Model file for the job. Use its own axes, mm. A direction names the side the tool comes from. Round coordinates to 2 decimals unless told otherwise and drop trailing zeros. Loops run counter-clockwise (first coordinate to the right, second up) from the corner with the lowest first, then second, coordinate; pieces in that order, holes last. Notation, with made-up numbers: (-7.75, -35) - (44.25, -35) arc R24 cw to (44.25, 0) - close; hole circle Ø7 at (81, 4.5). An arc over 180 degrees is marked (long way). Answer as a JSON object with one key per item and string values.
from build123d import *

# Parameters (mm, degrees)
RESSALTO_EXTRUS_O1_DEPTH = 65
ESBO_O2_W                = 40
ESBO_O2_H                = 40
RESSALTO_EXTRUS_O2_DEPTH = 4
ESBO_O4_W                = 5
ESBO_O4_H                = 5
RESSALTO_EXTRUS_O3_DEPTH = 13.5
ESBO_O5_W                = 40
ESBO_O5_H                = 40
ESBO_O5_W_2              = 30
ESBO_O5_H_2              = 30
RESSALTO_EXTRUS_O4_DEPTH = 4


with BuildPart() as part:
    # Esboço1 → Ressalto-extrusão1 (new body)
    with BuildSketch(Plane.XY):
        with BuildLine():
            Line((18, 0), (20, 0))
            Line((20, 0), (20, 40))
            Line((20, 40), (-20, 40))
            Line((-20, 40), (-20, 0))
            Line((-20, 0), (-18, 0))
            Line((-18, 0), (-18, 9))
            Line((-18, 9), (-18, 27))
            ThreePointArc((-18, 27), (-15.363961031, 33.363961031), (-9, 36))
            Line((-9, 36), (9, 36))
            ThreePointArc((9, 36), (15.363961031, 33.363961031), (18, 27))
            Line((18, 27), (18, 0))
        make_face()
    extrude(amount=RESSALTO_EXTRUS_O1_DEPTH)

    # Esboço2 → Ressalto-extrusão2 (add)
    with BuildSketch(Plane(origin=(0, 0, 0), x_dir=(-1, 0, 0), z_dir=(0, 0, -1))):
        with Locations((0, 20)):
            Rectangle(ESBO_O2_W, ESBO_O2_H)
        with BuildLine():
            Line((-5, 30), (-5, 6))
            ThreePointArc((-5, 6), (-9, 2), (-13, 6))
            Line((-13, 6), (-13, 30))
            ThreePointArc((-13, 30), (-9, 34), (-5, 30))
        make_face(mode=Mode.SUBTRACT)
        with BuildLine():
            Line((13, 30), (13, 6.321034479))
            ThreePointArc((13, 6.321034479), (9, 2.321034479), (5, 6.321034479))
            Line((5, 6.321034479), (5, 30))
            ThreePointArc((5, 30), (9, 34), (13, 30))
        make_face(mode=Mode.SUBTRACT)
    ressalto_extrus_o2 = extrude(amount=RESSALTO_EXTRUS_O2_DEPTH)

    # Esboço4 → Ressalto-extrusão3 (add)
    with BuildSketch(Plane(origin=(0, 0, -4), x_dir=(-1, 0, 0), z_dir=(0, 0, -1))):
        with Locations((17.5, 37.5)):
            Rectangle(ESBO_O4_W, ESBO_O4_H)
        with Locations((17.5, 2.5)):
            Rectangle(ESBO_O4_W, ESBO_O4_H)
        with Locations((-17.5, 37.5)):
            Rectangle(ESBO_O4_W, ESBO_O4_H)
        with Locations((-17.5, 2.5)):
            Rectangle(ESBO_O4_W, ESBO_O4_H)
    ressalto_extrus_o3 = extrude(amount=RESSALTO_EXTRUS_O3_DEPTH)

    # Esboço5 → Ressalto-extrusão4 (add)
    with BuildSketch(Plane(origin=(0, 0, -17.5), x_dir=(-1, 0, 0), z_dir=(0, 0, -1))):
        with Locations((0, 20)):
            Rectangle(ESBO_O5_W, ESBO_O5_H)
        with Locations((0, 20)):
            Rectangle(ESBO_O5_W_2, ESBO_O5_H_2, mode=Mode.SUBTRACT)
    ressalto_extrus_o4 = extrude(amount=RESSALTO_EXTRUS_O4_DEPTH)

    # Espelhar1: Ressalto-extrusão2, Ressalto-extrusão3, Ressalto-extrusão4 across plane
    add(ressalto_extrus_o2.mirror(Plane.XY.offset(32.5)))
    add(ressalto_extrus_o3.mirror(Plane.XY.offset(32.5)))
    add(ressalto_extrus_o4.mirror(Plane.XY.offset(32.5)))


solid = part.part
1) Tool access for faces 1 (the cylindrical face through (9, 34, 67)), 2 (the flat face through (0, 3, -17.5)), 3 (the flat face through (18, 14, 32)), 4 (the flat face through (-17, 35, 76)): list every direction of +Z, -Z, +X, -X, +Y, -Y with a clear straight run to the whole face (end or side of a thin tool).
Values follow:
{"face 1": "+Z, -Z", "face 2": "+Y, -Y", "face 3": "-Y", "face 4": "+X, -X"}
2) Slice it at C-C on x = -4. List the corners of the cut face in (y, z).
Values follow:
{"outline": "(0, -21.5) - (5, -21.5) - (5, -17.5) - (0, -17.5) - close; (0, -4) - (40, -4) - (40, 69) - (0, 69) - (0, 65) - (36, 65) - (36, 0) - (0, 0) - close; (0, 82.5) - (5, 82.5) - (5, 86.5) - (0, 86.5) - close; (35, -21.5) - (40, -21.5) - (40, -17.5) - (35, -17.5) - close; (35, 82.5) - (40, 82.5) - (40, 86.5) - (35, 86.5) - close"}
3) Slice it at D-D on z = 39. List the corners of the cut face in (x, y).
Values follow:
{"outline": "(-20, 0) - (-18, 0) - (-18, 27) arc R9 cw to (-9, 36) - (9, 36) arc R9 cw to (18, 27) - (18, 0) - (20, 0) - (20, 40) - (-20, 40) - close"}
4) Slice it at B-B on y = 37. List the corners of the cut face in (x, z).
Values follow:
{"outline": "(-20, -21.5) - (20, -21.5) - (20, 86.5) - (-20, 86.5) - close; hole (-15, -17.5) - (15, -17.5) - (15, -4) - (-15, -4) - close; hole (-15, 69) - (15, 69) - (15, 82.5) - (-15, 82.5) - close"}
5) Probe probe 1 along Z at (x, y) = (12, 36); probe 2 along Z at (x, y) = (-17.5, 8); probe 3 along Z at (x, y) = (13.5, 24.5). List the from-to ranges inside material, lowest first.
Values follow:
{"probe 1": "-21.5 to -17.5, -4 to 69, 82.5 to 86.5", "probe 2": "-21.5 to -17.5, -4 to 0, 65 to 69, 82.5 to 86.5", "probe 3": "-4 to 0, 65 to 69"}
6) Drop flat-ended pins along their axis: P1, Ø3, axis at x = 5.5, y = 19.5, coming from the +Z side; P2, Ø1, axis at x = 1, y = 21, coming from the -Z side. Give the stop position or say it passes through.
Values follow:
{"P1": "z = 69", "P2": "z = -4"}
7) Two-plate mould, pull along Y, no slides. Class faces 5 (the flat face through (0, 18, 65)), 6 (the cylindrical face through (15.294, 33.434, 32.045)), 7 (the flat face through (18, 5, 76)): pulls with the +Y half, pulls with the -Y half, needs draft (parallel to the pull), parting line crosses it, or undercut.
Values follow:
{"face 5": "needs draft", "face 6": "pulls with the -Y half", "face 7": "undercut"}
8) Slice it at A-A on z = -7.5. List the corners of the cut face in (x, y).
Values follow:
{"outline": "(-20, 0) - (-15, 0) - (-15, 5) - (-20, 5) - close; (-20, 35) - (-15, 35) - (-15, 40) - (-20, 40) - close; (15, 0) - (20, 0) - (20, 5) - (15, 5) - close; (15, 35) - (20, 35) - (20, 40) - (15, 40) - close"}
